from build123d import *

# Parameters (mm, degrees)
SKETCH1_R               = 4
BOSS_EXTRUDE1_DEPTH     = 12
SKETCH2_R               = 11
BOSS_EXTRUDE2_DEPTH     = 10
CUT_EXTRUDE1_DEPTH      = 20
CUT_EXTRUDE1_DEPTH_BACK = 20
SKETCH3_R               = 1.3


with BuildPart() as part:
    # Sketch1 → Boss-Extrude1 (new body)
    with BuildSketch(Plane.XY):
        Circle(SKETCH1_R)
    extrude(amount=BOSS_EXTRUDE1_DEPTH)

    # Sketch2 → Boss-Extrude2 (add)
    with BuildSketch(Plane(origin=(0, 0, 0), x_dir=(-1, 0, 0), z_dir=(0, 0, -1))):
        Circle(SKETCH2_R)
    extrude(amount=BOSS_EXTRUDE2_DEPTH)

    # Sketch3 → Cut-Extrude1 (cut, two sides: drawn at the far end of the back side and taken through both)
    with BuildSketch(Plane(origin=(0, 0, 0), x_dir=(1, 0, 0), z_dir=(0, 1, 0)).offset(-CUT_EXTRUDE1_DEPTH_BACK)):
        with Locations(Location((0, 4.2, 0), (0, 0, 90))):
            Circle(SKETCH3_R)
    extrude(amount=CUT_EXTRUDE1_DEPTH + CUT_EXTRUDE1_DEPTH_BACK, mode=Mode.SUBTRACT)


solid = part.part
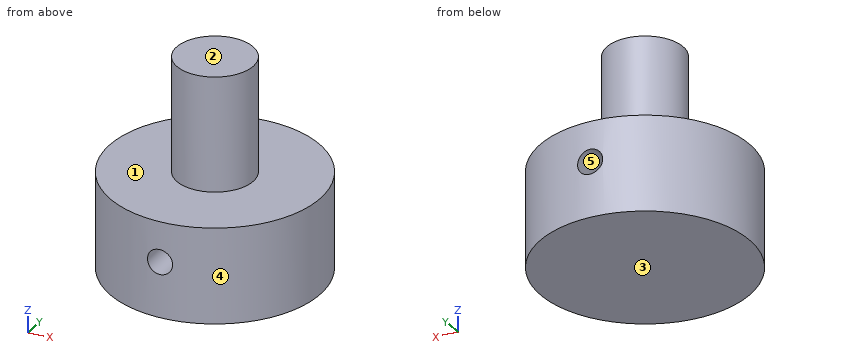
Design review of the part built by this model. Coordinates are the model's own, in mm. Face numbers are marked on the shaded views. A direction names the side the tool comes from. Give positions to 0.01 mm unless a question says otherwise; leave off trailing zeros. Order: outer loops, then holes, each group sorted by start corner. A loop starts at its lowest first (then second) coordinate and runs counter-clockwise, first axis right, second up. Notation, with made-up numbers: (-0.5, -4.5) - (25.5, -4.5) arc R20 ccw to (25.5, 30.5) - close; hole circle Ø8 at (12, 27.5). An arc over 180 degrees is marked (long way). Write item = value, one per line. Start each with the question number.
Q1. Tool access review of the marked faces 1 and 2: name each direction out of +Z, -Z, +X, -X, +Y, -Y from which nothing blocks a thin tool from reaching the whole face with its end or side.
Q2. We need section A-A on x = 0. State the section outline as (y, z) points, plus the area to 3 significant figures.
Q3. We need section D-D on z = -4.2. State the section outline as (x, y) points.
Q4. Mouldability with a two-part tool opening along X and no side actions: class the marked faces 3, 4 and 5 as released by +X, released by -X, zero draft, split by the parting line, or undercut.
Q5. Clearance check with flat-ended pins moving along their axes: pin 1 Ø5 at (x, z) = (-4.5, 5) entering from +Y; pin 2 Ø10 at (y, z) = (5.5, 1) entering from +X; pin 3 Ø1.5 at (x, z) = (-6.5, 7.5) entering from -Y; pin 4 Ø1 at (x, z) = (-1.5, 8) entering from -Y. State where each tip first meets the part, or that it passes through.
Q6. We need section B-B on y = 0. State the section outline as (x, z) points, plus the area to 3 significant figures.
Q7. We need section C-C on z = -1.25. State the section outline as (x, y) points, plus the area to 3 significant figures.
Q8. To check wall thickness, follow L1, parallel to Z at x = -6.5, y = 8.5; L2, parallel to X at y = -0.5, z = -4.2; L3, parallel to X at y = 4.75, z = -4.5. State the ranges of each line that lie inside material, in increasing order. Write a range as from..to.
Working result:
q1.face_1 = +Z
q1.face_2 = +Z, +X, -X, +Y, -Y
q2.outline = (-11, -10) - (11, -10) - (11, -5.5) - (-11, -5.5) - close; (-11, -2.9) - (11, -2.9) - (11, 0) - (4, 0) - (4, 12) - (-4, 12) - (-4, 0) - (-11, 0) - close
q2.area = 259 mm²
q3.outline = (-1.3, -10.92) - (-1.3, 10.92) arc R11 ccw to start; (1.3, -10.92) arc R11 ccw to (1.3, 10.92) - close
q4.face_3 = zero draft
q4.face_4 = split by the parting line
q4.face_5 = undercut
q5.pin_1 = 3.46
q5.pin_2 = 10.98
q5.pin_3 = through
q5.pin_4 = -3.87
q6.outline = (-11, -10) - (11, -10) - (11, 0) - (4, 0) - (4, 12) - (-4, 12) - (-4, 0) - (-11, 0) - close; hole circle Ø2.6 at (0, -4.2)
q6.area = 311 mm²
q7.outline = circle Ø22 at (0, 0)
q7.area = 380 mm²
q8.L1 = -10..0
q8.L2 = -10.99..-1.3, 1.3..10.99
q8.L3 = -9.92..-1.26, 1.26..9.92
